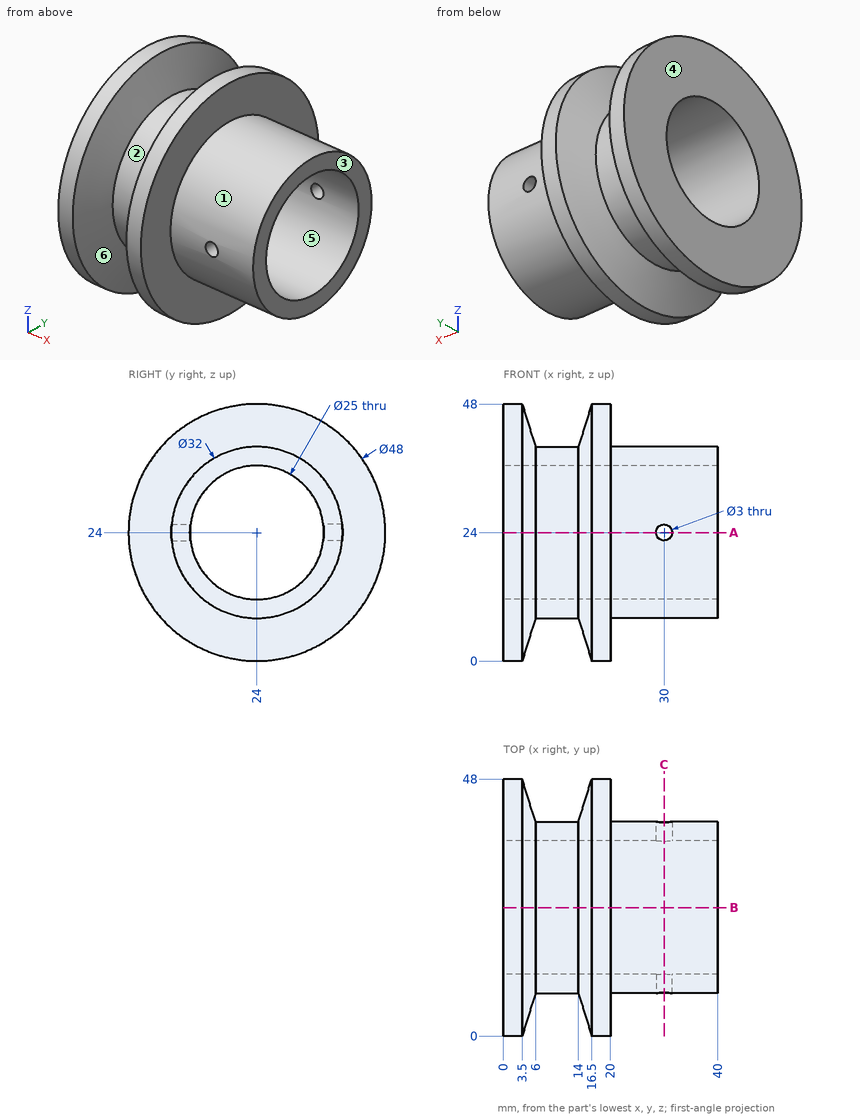
Input: dimensioned drawing with shaded views. Units: mm. Origin: part minimum x, y, z. A direction names the side the tool comes from. Coordinates: 2 decimals unless noted, no trailing zeros. Write each loop counter-clockwise with the first axis right and the second up, starting at its lowest first coordinate (ties: lowest second). Pieces come first, ordered by that corner, then holes. Notation, with made-up numbers: (6.5, 59) -> (37.5, 59) arc R16 cw to (37.5, 79) -> close; hole circle Ø10 at (37.5, 41). An arc over 180 degrees is marked (long way). Return JSON: item names as keys, results as strings. Group by question number.
1) Ray query, line 1 along Y through (x, z) = (12, 24); line 2 along X through (y, z) = (38, 24); line 3 along Z through (x, y) = (12.5, 14). Return the intervals inside material, ascending.
2) Section query B-B, the plane y = 24. Return loops of the section in (x, z).
3) Contact query for flat-ended pins moving along their axis: P1, Ø2, axis at x = 30.5, y = 26.5, coming from the -Z side; P2, Ø8, axis at x = 19.5, z = 41.5, coming from the +Y side; P3, Ø8, axis at x = 9.5, z = 39, coming from the -Y side. Output: stop coordinate, or through.
4) Section query A-A, the plane z = 24. Return loops of the section in (x, y), plus the area to 3 significant figures.
5) Section query C-C, the plane x = 30. Return loops of the section in (y, z), plus the area to 3 significant figures.
6) Set-up query: the marked faces 1, 2 and 3. Return all of +Z, -Z, +X, -X, +Y, -Y with unobstructed straight access to the full face (end or side cutting, diameter ignored); none if empty.
7) Mould query, pull axis Y, two halves, no side actions, for the marked faces 4, 5 and 6. Classes: +Y half, -Y half, draft (parallel to the pull), parting line (faces both ways), or undercut.
From the geometry:
{
 "1": {"line 1": "8 to 11.5, 36.5 to 40", "line 2": "0 to 28.5, 31.5 to 40", "line 3": "11.51 to 16.5, 31.5 to 36.49"},
 "2": {"outline": "(0, 0) -> (3.5, 0) -> (6, 8) -> (14, 8) -> (16.5, 0) -> (20, 0) -> (20, 8) -> (40, 8) -> (40, 11.5) -> (0, 11.5) -> close; (0, 36.5) -> (40, 36.5) -> (40, 40) -> (20, 40) -> (20, 48) -> (16.5, 48) -> (14, 40) -> (6, 40) -> (3.5, 48) -> (0, 48) -> close"},
 "3": {"P1": "z = 8.07", "P2": "y = 43.84", "P3": "y = 12.38"},
 "4": {"outline": "(0, 0) -> (3.5, 0) -> (6, 8) -> (14, 8) -> (16.5, 0) -> (20, 0) -> (20, 8) -> (28.5, 8) -> (28.5, 11.5) -> (0, 11.5) -> close; (0, 36.5) -> (28.5, 36.5) -> (28.5, 40) -> (20, 40) -> (20, 48) -> (16.5, 48) -> (14, 40) -> (6, 40) -> (3.5, 48) -> (0, 48) -> close; (31.5, 8) -> (40, 8) -> (40, 11.5) -> (31.5, 11.5) -> close; (31.5, 36.5) -> (40, 36.5) -> (40, 40) -> (31.5, 40) -> close", "area": "411 mm²"},
 "5": {"outline": "(8.07, 22.5) arc R16 ccw to (39.93, 22.5) -> (36.41, 22.5) arc R12.5 cw to (11.59, 22.5) -> close; (8.07, 25.5) -> (11.59, 25.5) arc R12.5 cw to (36.41, 25.5) -> (39.93, 25.5) arc R16 ccw to start", "area": "292 mm²"},
 "6": {"face 1": "+X", "face 2": "none", "face 3": "+Z, -Z, +X, +Y, -Y"},
 "7": {"face 4": "draft", "face 5": "undercut", "face 6": "parting line"}
}
